Geometry: final body of the model. Coordinates: model frame, mm. A direction names the side the tool comes from. Give positions to 0.01 mm unless a question says otherwise; leave off trailing zeros. Write each loop counter-clockwise with the first axis right and the second up, starting at its lowest first coordinate (ties: lowest second). Pieces come first, ordered by that corner, then holes. Notation, with made-up numbers: (-6, 88) -> (26, 88) arc R33 ccw to (26, 123) -> close; hole circle Ø1 at (-6, 79). An arc over 180 degrees is marked (long way). Answer in a Markdown table with one row per item. Add a question column.
Item 1: Access query for faces 4 (the flat face through (-5, 3, 0)), 5 (the cylindrical face through (1.617, -8.67, -1.726)), 6 (the flat face through (-5, 3, -3.5)). Directions: +Z, -Z, +X, -X, +Y, -Y. A direction counts if a zero-diameter tool reaches every point of the face in a straight line with its end or side. Return the directions, or none.
Item 2: Section query A-A on x = 0. Output: boundary loops of the cut face in (y, z), plus the area to 3 significant figures.
Item 3: Draft query along X for faces 1 (the cylindrical face through (-11, 0, -2)), 2 (the flat face through (6, 0, -2)), 3 (the cylindrical face through (-0.228, 9.735, -1.726)). Return one class per face: +X half, -X half, draft (parallel to the pull), parting line (faces both ways), or undercut.
Item 4: Section query D-D on z = -1.25. Output: boundary loops of the cut face in (x, y).
Item 5: Material intervals for probe 1 along Y at (x, z) = (0, -1.5); probe 2 along Y at (x, z) = (0, -7); probe 3 along Z at (x, y) = (-1.25, 5), sorted ascending. Write a range as from..to.
Item 6: Section query B-B on x = -8.75. Output: boundary loops of the cut face in (y, z), plus the area to 3 significant figures.
Item 7: First-contact query: P1, Ø4.5, axis at x = 0, y = -8, coming from the +Z side; P2, Ø3, axis at x = -7.5, z = -10.5, coming from the -Y side; P3, Ø5.5, axis at x = 0, y = 8, coming from the -Z side; P4, Ø1.5, axis at x = 3, z = -6.5, coming from the -Y side. Flat tips, straight axial feed; report the tip coordinate or a pass-through.
Item 8: Section query C-C on y = 2.25. Output: boundary loops of the cut face in (x, z).
```python
from build123d import *

# Parameters (mm, degrees)
SKETCH1_R                = 11
SKETCH1_R_2              = 5.1
SKETCH1_R_3              = 1.75
BOSS_EXTRUDE1_DEPTH      = 3.5
SKETCH2_R                = 5.1
SKETCH2_R_2              = 4
BOSS_EXTRUDE2_DEPTH      = 1.5
BOSS_EXTRUDE2_DEPTH_BACK = 13.5
CROQUIS1_W               = 13.137854129
CROQUIS1_H               = 23.868248077
CORTAR_EXTRUIR1_DEPTH    = 14.5


with BuildPart() as part:
    # Sketch1 → Boss-Extrude1 (new body)
    with BuildSketch(Plane.XY):
        Circle(SKETCH1_R)
        Circle(SKETCH1_R_2, mode=Mode.SUBTRACT)
        with Locations((0, 8)):
            Circle(SKETCH1_R_3, mode=Mode.SUBTRACT)
        with Locations((8, 0)):
            Circle(SKETCH1_R_3, mode=Mode.SUBTRACT)
        with Locations((0, -8)):
            Circle(SKETCH1_R_3, mode=Mode.SUBTRACT)
        with Locations((-8, 0)):
            Circle(SKETCH1_R_3, mode=Mode.SUBTRACT)
    extrude(amount=-BOSS_EXTRUDE1_DEPTH)

    # Sketch2 → Boss-Extrude2 (add, two sides)
    with BuildSketch(Plane.XY) as boss_extrude2_sk:
        Circle(SKETCH2_R)
        Circle(SKETCH2_R_2, mode=Mode.SUBTRACT)
    extrude(amount=BOSS_EXTRUDE2_DEPTH)
    extrude(boss_extrude2_sk.sketch, amount=-BOSS_EXTRUDE2_DEPTH_BACK)

    # Croquis1 → Cortar-Extruir1 (cut, through all)
    with BuildSketch(Plane.XY):
        with Locations((12.568927065, 0.450129168)):
            Rectangle(CROQUIS1_W, CROQUIS1_H)
    extrude(amount=-CORTAR_EXTRUIR1_DEPTH, mode=Mode.SUBTRACT)


solid = part.part
```
Findings below:
| question | item | result |
|---|---|---|
| 1 | face 4 | +Z |
| 1 | face 5 | +Z, -Z |
| 1 | face 6 | -Z |
| 2 | outline | (-11, -3.5) -> (-9.75, -3.5) -> (-9.75, 0) -> (-11, 0) -> close; (-6.25, -3.5) -> (-5.1, -3.5) -> (-5.1, -13.5) -> (-4, -13.5) -> (-4, 1.5) -> (-5.1, 1.5) -> (-5.1, 0) -> (-6.25, 0) -> close; (4, -13.5) -> (5.1, -13.5) -> (5.1, -3.5) -> (6.25, -3.5) -> (6.25, 0) -> (5.1, 0) -> (5.1, 1.5) -> (4, 1.5) -> close; (9.75, -3.5) -> (11, -3.5) -> (11, 0) -> (9.75, 0) -> close |
| 2 | area | 49.8 mm^2 |
| 3 | face 1 | parting line |
| 3 | face 2 | +X half |
| 3 | face 3 | undercut |
| 4 | outline | (6, -9.22) -> (6, 9.22) arc R11 ccw (long way) to start; hole circle Ø3.5 at (-8, 0); hole circle Ø8 at (0, 0); hole circle Ø3.5 at (0, -8); hole circle Ø3.5 at (0, 8) |
| 5 | probe 1 | y = -11..-9.75, -6.25..-4, 4..6.25, 9.75..11 |
| 5 | probe 2 | y = -5.1..-4, 4..5.1 |
| 5 | probe 3 | z = -3.5..0 |
| 6 | outline | (-6.67, -3.5) -> (-1.58, -3.5) -> (-1.58, 0) -> (-6.67, 0) -> close; (1.58, -3.5) -> (6.67, -3.5) -> (6.67, 0) -> (1.58, 0) -> close |
| 6 | area | 35.6 mm^2 |
| 7 | P1 | stops at z = 0 |
| 7 | P2 | passes through |
| 7 | P3 | stops at z = -3.5 |
| 7 | P4 | stops at y = -4.58 |
| 8 | outline | (-10.77, -3.5) -> (-4.58, -3.5) -> (-4.58, -13.5) -> (-3.31, -13.5) -> (-3.31, 1.5) -> (-4.58, 1.5) -> (-4.58, 0) -> (-10.77, 0) -> close; (3.31, -13.5) -> (4.58, -13.5) -> (4.58, -3.5) -> (6, -3.5) -> (6, 0) -> (4.58, 0) -> (4.58, 1.5) -> (3.31, 1.5) -> close |
